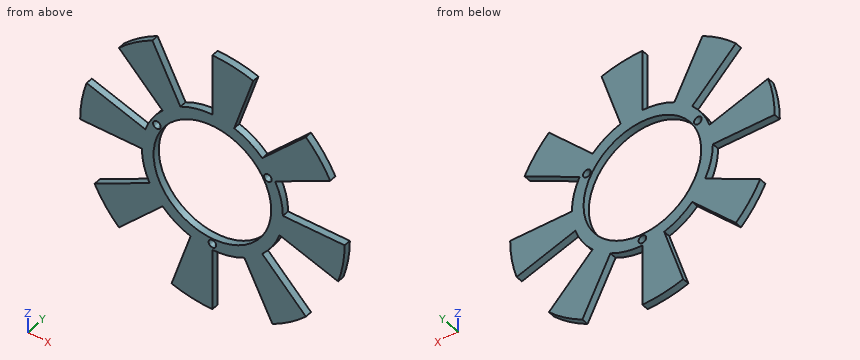
from build123d import *

# Parameters (mm, degrees)
SKETCH1_R           = 30.25
SKETCH1_R_2         = 25.25
EXTRUDE_THIN1_DEPTH = 3
SKETCH2_R           = 1.65
CUT_EXTRUDE3_DEPTH  = 10
BOSS_EXTRUDE1_DEPTH = 3


with BuildPart() as part:
    # Sketch1 → Extrude-Thin1 (new body)
    with BuildSketch(Plane(origin=(0, 0, 0), x_dir=(1, 0, 0), z_dir=(0, 1, 0))):
        Circle(SKETCH1_R)
        Circle(SKETCH1_R_2, mode=Mode.SUBTRACT)
    extrude(amount=-EXTRUDE_THIN1_DEPTH)

    # Sketch2 → Cut-Extrude3 (cut)
    with BuildSketch(Plane(origin=(0, 0, 0), x_dir=(1, 0, 0), z_dir=(0, 1, 0))):
        with Locations((0, 27.5)):
            Circle(SKETCH2_R)
        with Locations((23.815698604, -13.75)):
            Circle(SKETCH2_R)
        with Locations((-23.815698604, -13.75)):
            Circle(SKETCH2_R)
    extrude(amount=-CUT_EXTRUDE3_DEPTH, mode=Mode.SUBTRACT)

    # Sketch5 → Boss-Extrude1 (add)
    with BuildSketch(Plane.XZ.offset(3)):
        with BuildLine():
            Line((0, 56.75), (0, 30.25))
            ThreePointArc((0, 30.25), (4.732142567, 29.877572303), (9.34776408, 28.769459618))
            Line((9.34776408, 28.769459618), (17.536714431, 53.9724573))
            ThreePointArc((17.536714431, 53.9724573), (8.877655891, 56.051313329), (0, 56.75))
        make_face()
        with BuildLine():
            Line((40.128309832, 40.128309832), (21.389980131, 21.389980131))
            ThreePointArc((21.389980131, 21.389980131), (24.47276408, 17.780503882), (26.952947357, 13.733212617))
            Line((26.952947357, 13.733212617), (50.564620248, 25.76396086))
            ThreePointArc((50.564620248, 25.76396086), (45.911714431, 33.356813068), (40.128309832, 40.128309832))
        make_face()
        with BuildLine():
            Line((56.75, 0), (30.25, 0))
            ThreePointArc((30.25, 0), (29.877572303, -4.732142567), (28.769459618, -9.34776408))
            Line((28.769459618, -9.34776408), (53.9724573, -17.536714431))
            ThreePointArc((53.9724573, -17.536714431), (56.051313329, -8.877655891), (56.75, 0))
        make_face()
        with BuildLine():
            Line((40.128309832, -40.128309832), (21.389980131, -21.389980131))
            ThreePointArc((21.389980131, -21.389980131), (17.780503882, -24.47276408), (13.733212617, -26.952947357))
            Line((13.733212617, -26.952947357), (25.76396086, -50.564620248))
            ThreePointArc((25.76396086, -50.564620248), (33.356813068, -45.911714431), (40.128309832, -40.128309832))
        make_face()
        with BuildLine():
            Line((0, -56.75), (0, -30.25))
            ThreePointArc((0, -30.25), (-4.732142567, -29.877572303), (-9.34776408, -28.769459618))
            Line((-9.34776408, -28.769459618), (-17.536714431, -53.9724573))
            ThreePointArc((-17.536714431, -53.9724573), (-8.877655891, -56.051313329), (0, -56.75))
        make_face()
        with BuildLine():
            Line((-40.128309832, -40.128309832), (-21.389980131, -21.389980131))
            ThreePointArc((-21.389980131, -21.389980131), (-24.47276408, -17.780503882), (-26.952947357, -13.733212617))
            Line((-26.952947357, -13.733212617), (-50.564620248, -25.76396086))
            ThreePointArc((-50.564620248, -25.76396086), (-45.911714431, -33.356813068), (-40.128309832, -40.128309832))
        make_face()
        with BuildLine():
            Line((-56.75, 0), (-30.25, 0))
            ThreePointArc((-30.25, 0), (-29.877572303, 4.732142567), (-28.769459618, 9.34776408))
            Line((-28.769459618, 9.34776408), (-53.9724573, 17.536714431))
            ThreePointArc((-53.9724573, 17.536714431), (-56.051313329, 8.877655891), (-56.75, 0))
        make_face()
        with BuildLine():
            Line((-40.128309832, 40.128309832), (-21.389980131, 21.389980131))
            ThreePointArc((-21.389980131, 21.389980131), (-17.780503882, 24.47276408), (-13.733212617, 26.952947357))
            Line((-13.733212617, 26.952947357), (-25.76396086, 50.564620248))
            ThreePointArc((-25.76396086, 50.564620248), (-33.356813068, 45.911714431), (-40.128309832, 40.128309832))
        make_face()
    extrude(amount=-BOSS_EXTRUDE1_DEPTH)


solid = part.part
CAD build for the part. Positions are in the model's coordinates, mm. Coordinates: 2 decimals unless noted, no trailing zeros. Write each loop counter-clockwise with the first axis right and the second up, starting at its lowest first coordinate (ties: lowest second). Pieces come first, ordered by that corner, then holes. Notation, with made-up numbers: (3.25, 68.5) - (8.25, 68.5) arc R11 ccw to (8.25, 81.5) - close; hole circle Ø9 at (-2, -24.75). An arc over 180 degrees is marked (long way). Use a Markdown table: item, result. Add a question column.
Item 1: Band-saw the part on B-B, the plane x = 33. Give the cut face in (y, z), and give its area (3 significant figures).
Item 2: Drill centre lines: L1, parallel to X at y = -0.85, z = -26; L2, parallel to Z at x = -23, y = -0.15; L3, parallel to X at y = -2.3, z = -27.5. Where is each one in solid material? Low to high. Write a range as from..to.
Item 3: Band-saw the part on C-C, the plane y = -1.7. Give the number of separate pieces and of enclosed holes in the cut face, and give its area (3 significant figures).
Item 4: Band-saw the part on A-A, the plane z = -48.5. Give the cut face in (x, y).
Item 5: Flat gauge pins, fed straight in: pin 1 (3 mm diameter, centred on x = -38, z = 15.5, fed in from +Y); pin 2 (1 mm diameter, centred on y = -1, z = -39.5, fed in from -X); pin 3 (1 mm diameter, centred on x = 27, y = -0.5, fed in from -Z). Where does each tip first touch, or does it go through?
Item 6: Band-saw the part on D-D, the plane z = -7.5. Give the cut face in (x, y).
Numbers:
| question | item | result |
|---|---|---|
| 1 | outline | (-3, -46.17) - (0, -46.17) - (0, -33) - (-3, -33) - close; (-3, -10.72) - (0, -10.72) - (0, 0) - (-3, 0) - close; (-3, 16.81) - (0, 16.81) - (0, 33) - (-3, 33) - close |
| 1 | area | 120 mm2 |
| 2 | L1 | -50.44..-26, -15.46..-0.69, 0.69..26 |
| 2 | L2 | -23..-10.42, 10.42..12.32, 15.18..19.65, 23..45.14 |
| 2 | L3 | -49.64..-27.5, -12.6..-1.65, 1.65..12.6, 14.01..27.5 |
| 3 | separate pieces | 1 |
| 3 | enclosed holes | 4 |
| 3 | area | 3,740 mm2 |
| 4 | outline | (-15.76, -3) - (0, -3) - (0, 0) - (-15.76, 0) - close; (24.71, -3) - (29.47, -3) - (29.47, 0) - (24.71, 0) - close |
| 5 | pin 1 | through |
| 5 | pin 2 | x = -41.23 |
| 5 | pin 3 | z = -50.18 |
| 6 | outline | (-29.31, -3) - (-24.11, -3) - (-24.11, 0) - (-29.31, 0) - close; (24.11, -3) - (56.25, -3) - (56.25, 0) - (24.11, 0) - close |
